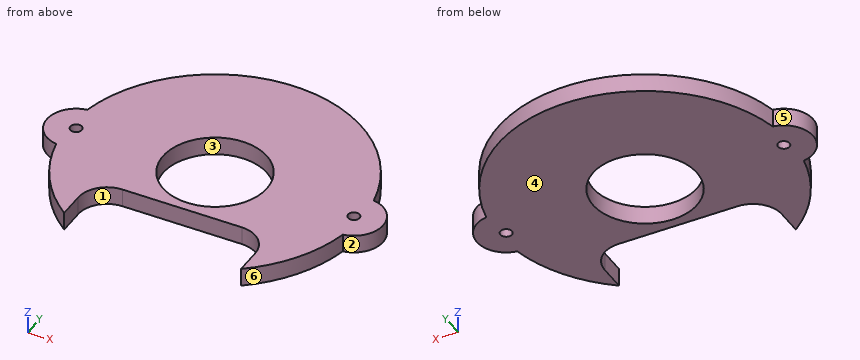
```python
from build123d import *

# Parameters (mm, degrees)
SKETCH1_R           = 1
SKETCH1_R_2         = 9
BOSS_EXTRUDE1_DEPTH = 3.175
CUT_EXTRUDE3_DEPTH  = 9.398
FILLET3_R           = 5


with BuildPart() as part:
    # Sketch1 → Boss-Extrude1 (new body)
    with BuildSketch(Plane.XY):
        with BuildLine():
            ThreePointArc((24.898684211, -5.021506207), (29.21, 0), (24.898684211, 5.021506207))
            ThreePointArc((24.898684211, 5.021506207), (0, 25.4), (-24.898684211, 5.021506207))
            ThreePointArc((-24.898684211, 5.021506207), (-29.21, 0), (-24.898684211, -5.021506207))
            ThreePointArc((-24.898684211, -5.021506207), (0, -25.4), (24.898684211, -5.021506207))
        make_face()
        with Locations((-24.13, 0)):
            Circle(SKETCH1_R, mode=Mode.SUBTRACT)
        with Locations((24.13, 0)):
            Circle(SKETCH1_R, mode=Mode.SUBTRACT)
        Circle(SKETCH1_R_2, mode=Mode.SUBTRACT)
    extrude(amount=BOSS_EXTRUDE1_DEPTH)

    # Sketch2 → Cut-Extrude3 (cut)
    with BuildSketch(Plane.XY):
        with BuildLine():
            Line((-15.367, -20.224126953), (-15.367, -10.654548843))
            Line((-15.367, -10.654548843), (15.367, -10.654548843))
            Line((15.367, -10.654548843), (15.367, -20.224126953))
            ThreePointArc((15.367, -20.224126953), (0, -25.4), (-15.367, -20.224126953))
        make_face()
    extrude(amount=CUT_EXTRUDE3_DEPTH, mode=Mode.SUBTRACT)

    # Fillet3
    fillet3_edges = [part.edges().sort_by_distance(p)[0] for p in [
        (15.367, -10.654548843, 1.5875),
        (-15.367, -10.654548843, 1.5875),
    ]]
    fillet(fillet3_edges, radius=FILLET3_R)


solid = part.part
```
Here's how the part is built. I have some questions about the finished solid (model axes, mm). Face numbers are marked on the shaded views. A direction names the side the tool comes from. Give positions to 0.01 mm unless a question says otherwise; leave off trailing zeros. Write each loop counter-clockwise with the first axis right and the second up, starting at its lowest first coordinate (ties: lowest second). Pieces come first, ordered by that corner, then holes. Notation, with made-up numbers: M 29.25,71.25 L 79.25,71.25 A19 cw 79.25,90.25 Z; hole C -23.5,27 d5. An arc over 180 degrees is marked long. Put each result on its own line as item: value. Start each with the question number.
Item 1: I need wall thicknesses on L1, parallel to Y at x = -25, z = 0.6; L2, parallel to X at y = -2, z = 2; L3, parallel to Y at x = -1.5, z = 0.75. Which ranges of each line are inside material? Lowest first, please. Write a range as from..to.
Item 2: If we section it at C-C, the plane x = 0: Write out the boundary of the cut face in (y, z) (3 decimals).
Item 3: If we section it at A-A, the plane z = 0.85: Write out the boundary of the cut face in (x, y), then the cut area to 3 significant figures.
Item 4: Will these pins go through, and if not, where does the flat tip stop? pin 1 (1.5 mm diameter, centred on y = -6, z = 1, fed in from +X); pin 2 (1.6 mm diameter, centred on x = -1, z = 2, fed in from -Y); pin 3 (1.6 mm diameter, centred on y = -17, z = 1, fed in from -X).
Item 5: On a 3-axis mill with a long thin cutter (end or side, diameter ignored), from which of +Z, -Z, +X, -X, +Y, -Y can I reach the whole of each face in a straight line? I mean the marked faces 1 and 2. Say none if no direction works.
Item 6: Thinking about a two-plate mould opening in X: for the marked faces 3, 4, 5 and 6, which applies, +X half, -X half, draft (parallel to the pull), parting line (faces both ways), or undercut?
Item 7: If we section it at D-D, the plane y = -11.5: Write out the boundary of the cut face in (x, z) (3 decimals).
Item 8: If we section it at B-B, the plane y = 0: Write out the boundary of the cut face in (x, z) (3 decimals).
Values:
1. L1: -5..-0.49, 0.49..5
1. L2: -28.8..-8.77, 8.77..28.8
1. L3: -10.65..-8.87, 8.87..25.36
2. outline: M -10.655,0 L -9,0 L -9,3.175 L -10.655,3.175 Z; M 9,0 L 25.4,0 L 25.4,3.175 L 9,3.175 Z
3. outline: M -24.9,-5.02 A25.4 ccw -15.37,-20.22 L -15.37,-15.65 A5 cw -10.37,-10.65 L 10.37,-10.65 A5 cw 15.37,-15.65 L 15.37,-20.22 A25.4 ccw 24.9,-5.02 A5.08 ccw 24.9,5.02 A25.4 ccw -24.9,5.02 A5.08 ccw Z; hole C -24.13,0 d2; hole C 0,0 d18; hole C 24.13,0 d2
3. area: 1,430 mm²
4. pin 1: x = 24.85
4. pin 2: y = -10.65
4. pin 3: x = -19.56
5. face 1: +Z, -Z, -Y
5. face 2: +Z, -Z, +X
6. face 3: undercut
6. face 4: draft
6. face 5: -X half
6. face 6: +X half
7. outline: M -22.648,0 L -13.149,0 L -13.149,3.175 L -22.648,3.175 Z; M 13.149,0 L 22.648,0 L 22.648,3.175 L 13.149,3.175 Z
8. outline: M -29.21,0 L -25.13,0 L -25.13,3.175 L -29.21,3.175 Z; M -23.13,0 L -9,0 L -9,3.175 L -23.13,3.175 Z; M 9,0 L 23.13,0 L 23.13,3.175 L 9,3.175 Z; M 25.13,0 L 29.21,0 L 29.21,3.175 L 25.13,3.175 Z
